The model under review builds one solid part; all positions refer to its coordinate system, in mm. Coordinates: 2 decimals unless noted, no trailing zeros. Loops run counter-clockwise (first coordinate to the right, second up) from the corner with the lowest first, then second, coordinate; pieces in that order, holes last. Notation, with made-up numbers: (-1.75, -4) - (6.25, -4) arc R10 ccw to (6.25, 12) - close; hole circle Ø4 at (42.25, 34.5). An arc over 180 degrees is marked (long way). Answer in a Markdown table with one row per item. Add a question column.
(1) We need section A-A on z = 0. Write out the cut boundary in (x, y) (3 decimals).
(2) We need section C-C on y = 1.6. Write out the cut boundary in (x, z), plus the area to 3 significant figures.
(3) For line 1 along X through (y, z) = (2, 0); line 2 along Z through (x, y) = (6.5, 2.55); line 3 along X through (y, z) = (1.55, 23.5), list the stretches that pass through material, from the lowest coordinate up.
(4) We need section B-B on x = 6.5. Write out the cut boundary in (y, z) (3 decimals), plus the area to 3 significant figures.
(5) Mouldability with a two-part tool opening along X and no side actions: class faces 1 (the cylindrical face through (21.4, 1.6, 9)), 2 (the cylindrical face through (-7.64, 1.61, -4.1)), 3 (the cylindrical face through (11.4, 1.57, -0.07)) as +X half, -X half, draft (parallel to the pull), parting line (faces both ways), or undercut.
(6) For P1, Ø1.8, axis at x = 6.5, z = 23.5, coming from the -Y side; P2, Ø4, axis at x = 8, z = 5.5, coming from the -Y side, all flat-tipped, find the tip position at first contact; note any pin that passes through.
(7) We need section D-D on z = 23.5. Write out the cut boundary in (x, y) (3 decimals).
from build123d import *

# Parameters (mm, degrees)
SKETCH1_W           = 30
SKETCH1_H           = 35
SKETCH1_R           = 1.6
BOSS_EXTRUDE1_DEPTH = 3.175
CUT_EXTRUDE1_REACH  = 5.175
SKETCH2_R           = 1
CUT_EXTRUDE2_DEPTH  = 4.175
FILLET1_R           = 3


with BuildPart() as part:
    # Sketch1 → Boss-Extrude1 (new body)
    with BuildSketch(Plane(origin=(0, 0, 0), x_dir=(1, 0, 0), z_dir=(0, 1, 0))):
        with Locations((6.5, -12.5)):
            Rectangle(SKETCH1_W, SKETCH1_H)
        Circle(SKETCH1_R, mode=Mode.SUBTRACT)
        with Locations((13, 0)):
            Circle(SKETCH1_R, mode=Mode.SUBTRACT)
    extrude(amount=BOSS_EXTRUDE1_DEPTH)

    # Sketch2 → Cut-Extrude1 (cut, up to next)
    with BuildSketch(Plane(origin=(0, 3.175, 0), x_dir=(1, 0, 0), z_dir=(0, 1, 0)), mode=Mode.PRIVATE) as cut_extrude1_sk1:
        with Locations((6.5, -23.5)):
            Circle(SKETCH2_R)
    cut_extrude1_tool1 = extrude(cut_extrude1_sk1.sketch, amount=-CUT_EXTRUDE1_REACH, mode=Mode.PRIVATE) & part.part
    add(cut_extrude1_tool1.solids().sort_by_distance((6.5, 3.175, 23.5))[0], mode=Mode.SUBTRACT)

    # Sketch3 → Cut-Extrude2 (cut, through all)
    with BuildSketch(Plane(origin=(0, 3.175, 0), x_dir=(1, 0, 0), z_dir=(0, 1, 0))):
        with BuildLine():
            Line((21.5, -9), (11.998845434, -26.5))
            ThreePointArc((11.998845434, -26.5), (6.5, -29.771562929), (1.001154566, -26.5))
            Line((1.001154566, -26.5), (-8.5, -9))
            Line((-8.5, -9), (-8.5, -30))
            Line((-8.5, -30), (21.5, -30))
            Line((21.5, -30), (21.5, -9))
        make_face()
    extrude(amount=-CUT_EXTRUDE2_DEPTH, mode=Mode.SUBTRACT)

    # Fillet1
    fillet1_edges = [part.edges().sort_by_distance(p)[0] for p in [
        (21.5, 1.5875, 9),
        (-8.5, 1.5875, 9),
        (-8.5, 1.5875, -5),
        (21.5, 1.5875, -5),
    ]]
    fillet(fillet1_edges, radius=FILLET1_R)


solid = part.part
Outcome:
| question | item | result |
|---|---|---|
| 1 | outline | (-8.5, 0) - (-1.6, 0) - (-1.6, 3.175) - (-8.5, 3.175) - close; (1.6, 0) - (11.4, 0) - (11.4, 3.175) - (1.6, 3.175) - close; (14.6, 0) - (21.5, 0) - (21.5, 3.175) - (14.6, 3.175) - close |
| 2 | outline | (-8.5, -2) arc R3 ccw to (-5.5, -5) - (18.5, -5) arc R3 ccw to (21.5, -2) - (21.5, 8.24) arc R3 ccw to (21.14, 9.67) - (12, 26.5) arc R6.26 ccw to (1, 26.5) - (-8.14, 9.67) arc R3 ccw to (-8.5, 8.24) - close; hole circle Ø3.2 at (0, 0); hole circle Ø2 at (6.5, 23.5); hole circle Ø3.2 at (13, 0) |
| 2 | area | 781 mm² |
| 3 | line 1 | -8.5 to -1.6, 1.6 to 11.4, 14.6 to 21.5 |
| 3 | line 2 | -5 to 22.5, 24.5 to 29.77 |
| 3 | line 3 | -0.63 to 5.5, 7.5 to 13.63 |
| 4 | outline | (0, -5) - (3.175, -5) - (3.175, 22.5) - (0, 22.5) - close; (0, 24.5) - (3.175, 24.5) - (3.175, 29.772) - (0, 29.772) - close |
| 4 | area | 104 mm² |
| 5 | face 1 | +X half |
| 5 | face 2 | -X half |
| 5 | face 3 | undercut |
| 6 | P1 | through |
| 6 | P2 | y = 0 |
| 7 | outline | (-0.628, 0) - (5.5, 0) - (5.5, 3.175) - (-0.628, 3.175) - close; (7.5, 0) - (13.628, 0) - (13.628, 3.175) - (7.5, 3.175) - close |
